```python
from build123d import *

# Parameters (mm, degrees)
SKETCH_1_W          = 147
SKETCH_1_H          = 82
SKETCH_1_R          = 1.5
EXTRUDE_1_DEPTH     = 3
SKETCH_2_R          = 1.5
CUT_EXTRUDE_1_DEPTH = 3


with BuildPart() as part:
    # 草图1 → 凸台-拉伸1 (new body)
    with BuildSketch(Plane.XY):
        with Locations((-3.474545455, -5.452727273)):
            Rectangle(SKETCH_1_W, SKETCH_1_H)
        with Locations((-70.974545455, 29.547272727)):
            Circle(SKETCH_1_R, mode=Mode.SUBTRACT)
        with Locations(Location((64.025454545, 29.547272727, 0), (0, 0, 180))):
            Circle(SKETCH_1_R, mode=Mode.SUBTRACT)
        with Locations((64.025454545, -40.452727273)):
            Circle(SKETCH_1_R, mode=Mode.SUBTRACT)
        with Locations(Location((-70.974545455, -40.452727273, 0), (0, 0, 180))):
            Circle(SKETCH_1_R, mode=Mode.SUBTRACT)
    extrude(amount=EXTRUDE_1_DEPTH)

    # 草图2 → 切除-拉伸1 (cut)
    with BuildSketch(Plane(origin=(0, 0, 0), x_dir=(-1, 0, 0), z_dir=(0, 0, -1))):
        with Locations((-55.025454545, 14.547272727)):
            Circle(SKETCH_2_R)
        with Locations((-55.025454545, -25.452727273)):
            Circle(SKETCH_2_R)
        with Locations((61.974545455, -25.452727273)):
            Circle(SKETCH_2_R)
        with Locations((61.974545455, 14.547272727)):
            Circle(SKETCH_2_R)
    extrude(amount=-CUT_EXTRUDE_1_DEPTH, mode=Mode.SUBTRACT)


solid = part.part
```
Input: part model. Units: mm. Frame: model coordinates. Coordinates: 2 decimals unless noted, no trailing zeros. Answer in a Markdown table with one row per item.
(1) Mould query, pull axis Y, two halves, no side actions, for faces 1 (the face through (-5, -5, 3)), 2 (the face through (63.22, 28.28, 1.48)), 3 (the face through (-5, 35.547, 1)), 4 (the face through (-5, -46.453, 1)). Classes: pulls with the +Y half, pulls with the -Y half, needs draft (parallel to the pull), parting line crosses it, or undercut.
Model answer:
| item | result |
|---|---|
| face 1 | needs draft |
| face 2 | undercut |
| face 3 | pulls with the +Y half |
| face 4 | pulls with the -Y half |
(2) Material intervals for L1, parallel to X at y = 29, z = 0.3; L2, parallel to X at y = 14, z = 1.2; L3, parallel to Y at x = 56, z = 1.6, sorted ascending. Write a range as from..to.
Model answer:
| item | result |
|---|---|
| L1 | x = -76.97..-72.37, -69.58..62.63, 65.42..70.03 |
| L2 | x = -76.97..-63.37, -60.58..53.63, 56.42..70.03 |
| L3 | y = -46.45..-26.59, -24.31..13.41, 15.69..35.55 |
(3) Pin query (flat end, axial travel): P1, Ø5, axis at x = 55.03, y = -25.45, coming from the -Z side. Return the tip coordinate at first contact, or that it passes through.
Model answer:
| item | result |
|---|---|
| P1 | stops at z = 0 |
